Can you work these out from the model? Positions are in its coordinate system, mm. Face numbers are marked on the shaded views. Coordinates: 2 decimals unless noted, no trailing zeros. Loops run counter-clockwise (first coordinate to the right, second up) from the corner with the lowest first, then second, coordinate; pieces in that order, holes last.
```python
from build123d import *

# Parameters (mm, degrees)
SKETCH2_W           = 40
SKETCH2_H           = 40
SKETCH2_R           = 5
SKETCH2_R_2         = 11
BOSS_EXTRUDE1_DEPTH = 15
SKETCH3_R           = 5.1
CUT_EXTRUDE1_DEPTH  = 48.16990566


with BuildPart() as part:
    # Sketch2 → Boss-Extrude1 (new body)
    with BuildSketch(Plane.XY):
        Rectangle(SKETCH2_W, SKETCH2_H)
        with Locations((12, 7)):
            Circle(SKETCH2_R, mode=Mode.SUBTRACT)
        with Locations((-7, 7)):
            Circle(SKETCH2_R_2, mode=Mode.SUBTRACT)
    extrude(amount=BOSS_EXTRUDE1_DEPTH)

    # Sketch3 → Cut-Extrude1 (cut, through all)
    with BuildSketch(Plane(origin=(20, 0, 0), x_dir=(0, 0, -1), z_dir=(1, 0, 0))):
        with Locations((-7.5, -13)):
            Circle(SKETCH3_R)
    extrude(amount=-CUT_EXTRUDE1_DEPTH, mode=Mode.SUBTRACT)


solid = part.part
```
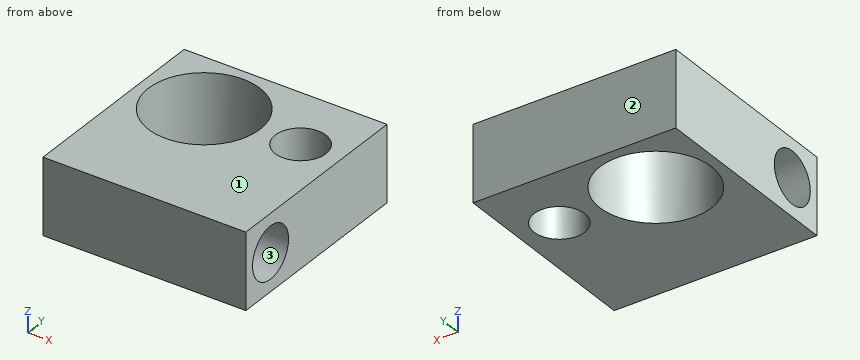
(1) If we mould it in two halves opening along Y, with no side actions, what happens to the marked faces 1, 2 and 3? For each: released by +Y, released by -Y, zero draft, split by the parting line, or undercut.
Check values:
face 1: zero draft
face 2: released by +Y
face 3: undercut
(2) I want a section at D-D on z = 1.25. Write out the boundary of the cut face in (x, y).
Check values:
outline: (-20, -20) - (20, -20) - (20, 20) - (-20, 20) - close; hole circle Ø22 at (-7, 7); hole circle Ø10 at (12, 7)
(3) I want a section at C-C on z = 7.5. Write out the boundary of the cut face in (x, y), then the cut area to 3 significant figures.
Check values:
outline: (-20, -20) - (20, -20) - (20, -18.1) - (-20, -18.1) - close; (-20, -7.9) - (20, -7.9) - (20, 20) - (-20, 20) - close; hole circle Ø22 at (-7, 7); hole circle Ø10 at (12, 7)
area: 733 mm2
(4) If I drill on probe 1 along Y at (x, z) = (12, 11.75); probe 2 along Y at (x, z) = (-7, 11.75); probe 3 along X at (y, z) = (14, 8), over which ranges is the centre line in solid material (lowest first)?
Check values:
probe 1: y = -20 to -15.82, -10.18 to 2, 12 to 20
probe 2: y = -20 to -15.82, -10.18 to -4, 18 to 20
probe 3: x = -20 to -15.49, 1.49 to 20
(5) I want a section at A-A on x = -7. Write out the boundary of the cut face in (y, z), then the cut area to 3 significant figures.
Check values:
outline: (-20, 0) - (-4, 0) - (-4, 15) - (-20, 15) - close; (18, 0) - (20, 0) - (20, 15) - (18, 15) - close; hole circle Ø10.2 at (-13, 7.5)
area: 188 mm2
(6) I want a section at B-B on y = 7. Write out the boundary of the cut face in (x, z).
Check values:
outline: (-20, 0) - (-18, 0) - (-18, 15) - (-20, 15) - close; (4, 0) - (7, 0) - (7, 15) - (4, 15) - close; (17, 0) - (20, 0) - (20, 15) - (17, 15) - close
